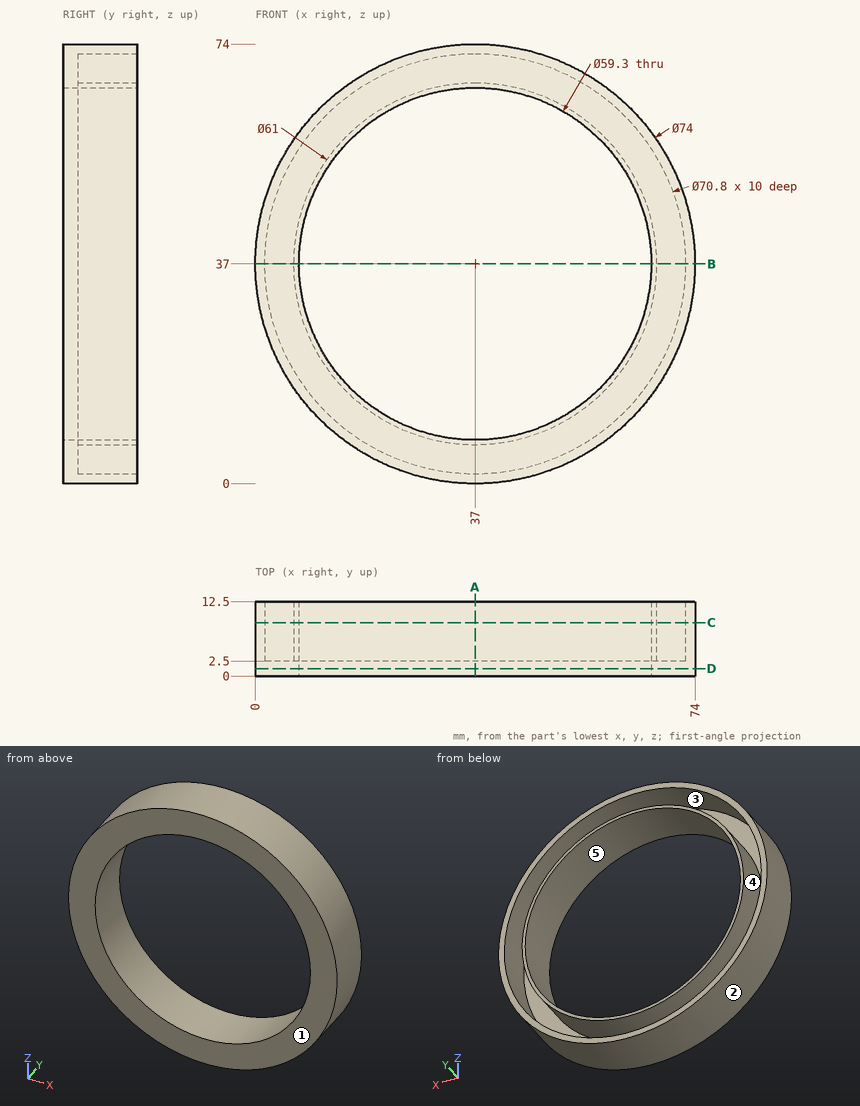
Answer from the drawing. Dimensions are ordinates in mm from the lowest x, y and z of the part. A direction names the side the tool comes from. Give positions to 0.01 mm unless a question says otherwise; leave off trailing zeros. Order: outer loops, then holes, each group sorted by start corner. A loop starts at its lowest first (then second) coordinate and runs counter-clockwise, first axis right, second up.
(1) Find section D-D (y = 1.25). Give the vertices of the cut face in (x, z).
(2) Straight lines are drawn through the part: L1, parallel to X at y = 6.5, z = 37; L2, parallel to X at y = 7.25, z = 26; L3, parallel to Z at x = 56.5, y = 3.25. For each, find the intervals that lie inside material, in ascending order.
(3) Find section A-A (x = 37). Give the vertices of the cut face in (y, z), plus the area to 4 significant figures.
(4) Given pin 1 (2 mm diameter, centred on x = 42, y = 8, fed in from -Z); pin 2 (3 mm diameter, centred on y = 4, z = 51, fed in from +X); pin 3 (4 mm diameter, centred on x = 38.5, y = 6.5, fed in from +Z); pin 4 (2 mm diameter, centred on y = 5.5, z = 15.5, fed in from +X), each flat-ended and moving along its own axis, determine where each tip first touches the part or whether it passes through.
(5) Find section B-B (z = 37). Give the vertices of the cut face in (x, y).
(6) For a pull along X with two mould halves and no side action, classify the marked faces 1, 2 and 3 as released by +X, released by -X, zero draft, split by the parting line, or undercut.
(7) For the marked faces 4 and 5, determine the directions among +Z, -Z, +X, -X, +Y, -Y from which every point of the face is accessible in a straight line to the end or side of a thin tool.
(8) Find section C-C (y = 9). Give the vertices of the cut face in (x, z).
Result sheet:
1. outline: circle Ø74 at (37, 37); hole circle Ø59.3 at (37, 37)
2. L1: x = 0 to 1.6, 6.5 to 7.35, 66.65 to 67.5, 72.4 to 74
2. L2: x = 1.67 to 3.35, 8.55 to 9.47, 64.53 to 65.45, 70.65 to 72.33
2. L3: z = 5.56 to 7.45, 13.55 to 14.66, 59.34 to 60.45, 66.55 to 68.44
3. outline: (0, 0) - (12.5, 0) - (12.5, 1.6) - (2.5, 1.6) - (2.5, 6.5) - (12.5, 6.5) - (12.5, 7.35) - (0, 7.35) - close; (0, 66.65) - (12.5, 66.65) - (12.5, 67.5) - (2.5, 67.5) - (2.5, 72.4) - (12.5, 72.4) - (12.5, 74) - (0, 74) - close
3. area: 85.75 mm2
4. pin 1: stops at z = 0.22
4. pin 2: stops at x = 71.82
4. pin 3: stops at z = 74
4. pin 4: stops at x = 67.8
5. outline: (0, 0) - (7.35, 0) - (7.35, 12.5) - (6.5, 12.5) - (6.5, 2.5) - (1.6, 2.5) - (1.6, 12.5) - (0, 12.5) - close; (66.65, 0) - (74, 0) - (74, 12.5) - (72.4, 12.5) - (72.4, 2.5) - (67.5, 2.5) - (67.5, 12.5) - (66.65, 12.5) - close
6. face 1: zero draft
6. face 2: split by the parting line
6. face 3: undercut
7. face 4: +Y
7. face 5: +Y, -Y
8. outline: circle Ø74 at (37, 37); circle Ø61 at (37, 37); hole circle Ø70.8 at (37, 37); hole circle Ø59.3 at (37, 37)
